from build123d import *

# Parameters (mm, degrees)
EXTRUDE_1_DEPTH            = 25
SKETCH_4_R                 = 22
CUT_EXTRUDE_1_DEPTH        = 1.8
CUT_EXTRUDE_START          = 6
CUT_EXTRUDE_1_2_DEPTH      = 3
SKETCH_11_W                = 19
SKETCH_11_H                = 1.4
EXTRUDE_3_DEPTH            = 1.5
FILLET_1_R                 = 0.25
SKETCH_14_W                = 0.8
SKETCH_14_H                = 6.2
CUT_EXTRUDE_2_DEPTH        = 1
CUT_EXTRUDE_1_3_REACH      = 110.009
CUT_EXTRUDE_1_3_END_RADIUS = 11.2
SKETCH_15_W                = 2.85
SKETCH_15_H                = 12
FILLET_1_2_R               = 1
CUT_EXTRUDE_2_2_REACH      = 94.909
SKETCH_16_R                = 1


with BuildPart() as part:
    # 草图2 → 整体拉伸-薄壁1 (new, symmetric)
    with BuildSketch(Plane.XY):
        with BuildLine():
            Line((29.091335385, 6.904737634), (30.691335385, 6.904737634))
            ThreePointArc((30.691335385, 6.904737634), (38.882855828, 11.16897327), (40.088261593, 20.324939067))
            Line((40.088261593, 20.324939067), (11.65650271, 98.440554593))
            Line((11.65650271, 98.440554593), (14.475580572, 99.466615023))
            Line((14.475580572, 99.466615023), (42.907339455, 21.350999497))
            ThreePointArc((42.907339455, 21.350999497), (41.340311961, 9.448243961), (30.691335385, 3.904737634))
            Line((30.691335385, 3.904737634), (29.091335385, 3.904737634))
            Line((29.091335385, 3.904737634), (29.091335385, 6.904737634))
        make_face()
    extrude(amount=EXTRUDE_1_DEPTH, both=True)

    # 草图4 → Cut-Extrude 1 (cut)
    with BuildSketch(Plane(origin=(44.750213172, 16.287745572, 0), x_dir=(0, 0, -1), z_dir=(0.9396926207859071, 0.3420201433256726, 0))):
        with Locations(Location((0, 63.117104009, 0), (0, 0, 90))):
            Circle(SKETCH_4_R)
    extrude(amount=-CUT_EXTRUDE_1_DEPTH, mode=Mode.SUBTRACT)

    # 草图3 → Cut-Extrude 1 2 (cut)
    with BuildSketch(Plane.XY.offset(CUT_EXTRUDE_START)):
        with BuildLine():
            ThreePointArc((29.091335385, 5.819612465), (39.382240762, 9.840166611), (41.215892738, 20.735363239))
            Line((41.215892738, 20.735363239), (28.995888649, 54.30954854))
            Line((28.995888649, 54.30954854), (27.969828219, 57.128626402))
            Line((27.969828219, 57.128626402), (29.661274936, 57.74426266))
            Line((29.661274936, 57.74426266), (30.687335366, 54.925184798))
            Line((30.687335366, 54.925184798), (42.907339455, 21.350999497))
            ThreePointArc((42.907339455, 21.350999497), (40.778993412, 8.704789126), (28.834192528, 4.038074492))
            Line((28.834192528, 4.038074492), (29.091335385, 5.819612465))
        make_face()
    cut_extrude_1_2 = extrude(amount=-CUT_EXTRUDE_1_2_DEPTH, mode=Mode.SUBTRACT)

    # 镜向1: Cut-Extrude 1 2 across plane
    add(cut_extrude_1_2.mirror(Plane.XY), mode=Mode.SUBTRACT)

    # 草图11 → 底部卡扣凸台-拉伸3 (add)
    with BuildSketch(Plane.ZY.offset(-29.091335385)):
        with Locations((-15.5, 4.604737634)):
            Rectangle(SKETCH_11_W, SKETCH_11_H)
        with Locations((15.5, 4.604737634)):
            Rectangle(SKETCH_11_W, SKETCH_11_H)
    extrude(amount=EXTRUDE_3_DEPTH)

    # Fillet 1
    fillet_1_edges = [part.edges().sort_by_distance(p)[0] for p in [
        (27.591335385, 4.604737634, 6),
        (27.591335385, 3.904737634, 15.5),
        (27.591335385, 4.604737634, 25),
        (27.591335385, 5.304737634, 15.5),
        (27.591335385, 4.604737634, -25),
        (27.591335385, 3.904737634, -15.5),
        (27.591335385, 4.604737634, -6),
        (27.591335385, 5.304737634, -15.5),
    ]]
    fillet(fillet_1_edges, radius=FILLET_1_R)

    # 草图14 → Cut-Extrude 2 (cut)
    with BuildSketch(Plane(origin=(-30.2746326, 83.178869451, 0), x_dir=(0.9396926207859067, 0.3420201433256736, 0), z_dir=(-0.3420201433256736, 0.9396926207859068, 0))):
        with Locations((46.022182172, 0)):
            Rectangle(SKETCH_14_W, SKETCH_14_H)
    extrude(amount=-CUT_EXTRUDE_2_DEPTH, mode=Mode.SUBTRACT)

    # Cut-Extrude 1 3: up to this cylinder (the profile starts outside it)
    cut_extrude_1_3_end = Plane(origin=(30.691335385, 16.904737634, 0), z_dir=(0, 0, 1)) * Cylinder(CUT_EXTRUDE_1_3_END_RADIUS, 243.418, mode=Mode.PRIVATE)
    # 草图15 → Cut-Extrude 1 3 (cut, up to the surface)
    with BuildSketch(Plane.XZ.offset(-3.904737634), mode=Mode.PRIVATE) as cut_extrude_1_3_sk1:
        with Locations((29.266335385, 0)):
            Rectangle(SKETCH_15_W, SKETCH_15_H)
    cut_extrude_1_3_tool1 = extrude(cut_extrude_1_3_sk1.sketch, amount=-CUT_EXTRUDE_1_3_REACH, mode=Mode.PRIVATE) - cut_extrude_1_3_end
    add(cut_extrude_1_3_tool1.solids().sort_by_distance((29.266335, 3.904738, 0))[0], mode=Mode.SUBTRACT)

    # Fillet 1 2
    fillet_1_2_edges = [part.edges().sort_by_distance(p)[0] for p in [
        (30.691335385, 3.904737634, 0),
        (36.762193938, 38.234648046, 3),
        (41.340311961, 9.448243961, 3),
        (41.340311961, 9.448243961, -3),
        (36.762193938, 38.234648046, -3),
    ]]
    fillet(fillet_1_2_edges, radius=FILLET_1_2_R)

    # 草图16 → Cut-Extrude 2 2 (cut, up to next)
    with BuildSketch(Plane(origin=(41.93113531, 15.261685142, 0), x_dir=(0, 0, 1), z_dir=(-0.9396926207859069, -0.3420201433256731, 0)), mode=Mode.PRIVATE) as cut_extrude_2_2_sk1:
        with Locations(Location((-22.5, 82.017104009, 0), (0, 0, 270))):
            Circle(SKETCH_16_R)
    cut_extrude_2_2_tool1 = extrude(cut_extrude_2_2_sk1.sketch, amount=-CUT_EXTRUDE_2_2_REACH, mode=Mode.PRIVATE) & part.part
    # 草图16 → Cut-Extrude 2 2 (cut, up to next)
    with BuildSketch(Plane(origin=(41.93113531, 15.261685142, 0), x_dir=(0, 0, 1), z_dir=(-0.9396926207859069, -0.3420201433256731, 0)), mode=Mode.PRIVATE) as cut_extrude_2_2_sk2:
        with Locations(Location((22.5, 82.017104009, 0), (0, 0, 270))):
            Circle(SKETCH_16_R)
    cut_extrude_2_2_tool2 = extrude(cut_extrude_2_2_sk2.sketch, amount=-CUT_EXTRUDE_2_2_REACH, mode=Mode.PRIVATE) & part.part
    add(cut_extrude_2_2_tool1.solids().sort_by_distance((13.879634, 92.332553, -22.5))[0], mode=Mode.SUBTRACT)
    add(cut_extrude_2_2_tool2.solids().sort_by_distance((13.879634, 92.332553, 22.5))[0], mode=Mode.SUBTRACT)


solid = part.part
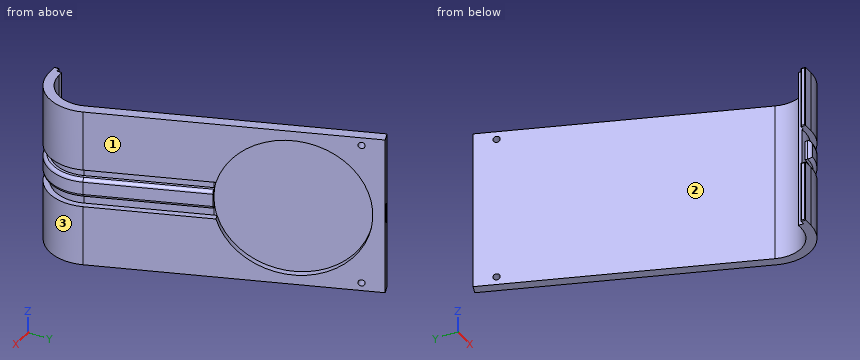
Input: part model. Units: mm. Frame: model coordinates. Face numbers are marked on the shaded views. Coordinates: 2 decimals unless noted, no trailing zeros. Order: outer loops, then holes, each group sorted by start corner. A loop starts at its lowest first (then second) coordinate and runs counter-clockwise, first axis right, second up. Notation, with made-up numbers: M -38,-3.75 L -32,-3.75 A12 ccw -32,1.25 Z; hole C 18,77 d2. An arc over 180 degrees is marked long. Answer in a Markdown table with one row per item.
(1) Draft query along Y for the marked faces 1, 2 and 3. Return one class per face: pulls with the +Y half, pulls with the -Y half, needs draft (parallel to the pull), parting line crosses it, or undercut.
Numbers:
| item | result |
|---|---|
| face 1 | pulls with the +Y half |
| face 2 | undercut |
| face 3 | parting line crosses it |
(2) Section query A-A, the plane z = 5. Output: boundary loops of the cut face in (x, y).
Numbers:
| item | result |
|---|---|
| outline | M 11.66,98.44 L 40.09,20.32 A10 cw 30.69,6.9 L 29.09,6.9 L 29.09,5.82 A11.2 ccw 41.22,20.74 L 14.14,95.12 L 15.84,95.73 L 14.48,99.47 Z |
(3) Section query D-D, the plane z = -11. Output: boundary loops of the cut face in (x, y).
Numbers:
| item | result |
|---|---|
| outline | M 11.66,98.44 L 40.09,20.32 A10 cw 30.69,6.9 L 29.09,6.9 L 29.09,5.3 L 27.84,5.3 A0.25 ccw 27.59,5.05 L 27.59,4.15 A0.25 ccw 27.84,3.9 L 30.69,3.9 A13 ccw 42.91,21.35 L 29.68,57.69 L 27.99,57.08 L 14.96,92.89 L 16.65,93.5 L 14.48,99.47 Z |
(4) Material intervals for line 1 (Z direction, x = 37, y = 35); line 2 (X direction, y = 17.5, z = 1.5); line 3 (X direction, y = 52.5, z = -21), sorted ascending. Write a range as [from, to].
Numbers:
| item | result |
|---|---|
| line 1 | z = [-25, -6], [-2.99, 2.99], [6, 25] |
| line 2 | x = [40.67, 43.68] |
| line 3 | x = [28.38, 31.57] |
(5) Contact query for flat-ended pins moving along their axis: pin 1 Ø0.6 at (x, z) = (28, -15.5) entering from +Y; pin 2 Ø0.5 at (y, z) = (4.5, -11.5) entering from -X; pin 3 Ø1.8 at (y, z) = (6, 2) entering from -X; pin 4 Ø10 at (x, z) = (27, 5.5) entering from -Y. Output: stop coordinate, or through.
Numbers:
| item | result |
|---|---|
| pin 1 | stops at y = 61.09 |
| pin 2 | stops at x = 27.59 |
| pin 3 | stops at x = 29.09 |
| pin 4 | stops at y = 3.9 |
(6) Section query B-B, the plane z = 16. Output: boundary loops of the cut face in (x, y), plus the area to 3 significant figures.
Numbers:
| item | result |
|---|---|
| outline | M 11.66,98.44 L 40.09,20.32 A10 cw 30.69,6.9 L 29.09,6.9 L 29.09,5.3 L 27.84,5.3 A0.25 ccw 27.59,5.05 L 27.59,4.15 A0.25 ccw 27.84,3.9 L 30.69,3.9 A13 ccw 42.91,21.35 L 28.33,61.41 L 26.64,60.79 L 16.31,89.17 L 18,89.79 L 14.48,99.47 Z |
| area | 268 mm^2 |
(7) Section query C-C, the plane x = 16. Give the number of separate pieces and of enclosed holes in the cut face, plus the area to 3 significant figures.
Numbers:
| item | result |
|---|---|
| separate pieces | 1 |
| enclosed holes | 2 |
| area | 309 mm^2 |
